Input: part model. Units: mm. Frame: model coordinates. A direction names the side the tool comes from. Round coordinates to 2 decimals unless told otherwise and drop trailing zeros. Loops run counter-clockwise (first coordinate to the right, second up) from the corner with the lowest first, then second, coordinate; pieces in that order, holes last. Notation, with made-up numbers: (51, 6.5) -> (76, 6.5) arc R19 cw to (76, 28.5) -> close; hole circle Ø5 at (66, 22). An arc over 180 degrees is marked (long way). Answer in a Markdown table with one row per item. Add a question column.
Q1. Reachability of faces 5 (the face through (0, -14, 7.7)), 6 (the face through (0, -5.76, 7)), 7 (the face through (7, 15.24, 7)), 8 (the face through (19, -13.502, 5)), 9 (the face through (-19, 1.102, 5)) from +Z, -Z, +X, -X, +Y, -Y: full face, straight path, thin tool, end or side. Return the list, or none.
Q2. Section D-D, the plane z = 11. Output: boundary loops of the cut face in (x, y), and give its area (3 significant figures).
Q3. Section A-A, the plane x = 22. Output: boundary loops of the cut face in (y, z), and give its area (3 significant figures).
Q4. Ray query, L1, parallel to X at y = 1.5, z = 3.75; L2, parallel to Y at x = -22, z = 1.25; L3, parallel to X at y = -10.5, z = 6.75. Return the intervals inside material, ascending. Write a range as from..to.
Q5. Pin query (flat end, axial travel): pin 1 (3 mm diameter, centred on x = 19.5, z = 6, fed in from +Y); pin 2 (6.5 mm diameter, centred on x = 22, z = 6, fed in from -Y); pin 3 (0.7 mm diameter, centred on y = 15.5, z = 7.5, fed in from -X); pin 4 (2.5 mm diameter, centred on x = 22, y = 17, fed in from +Z). Return the tip coordinate at first contact, or that it passes through.
Q6. Mould query, pull axis X, two halves, no side actions, for faces 1 (the face through (4.5, 16, 7)), 2 (the face through (-19, -13.502, 5)), 3 (the face through (13.5, 7, 5)), 4 (the face through (6.2, -14, 5)). Classes: pulls with the +X half, pulls with the -X half, needs draft (parallel to the pull), parting line crosses it, or undercut.
Q7. Section C-C, the plane y = -17. Output: boundary loops of the cut face in (x, z).
Q8. Section B-B, the plane z = 4.25. Output: boundary loops of the cut face in (x, y), and give its area (3 significant figures).
Autodesk Inventor part; units mm, degrees
ref_plane "YZ Plane" through (0, 0, 0) normal (1, 0, 0) x (0, 1, 0)
ref_plane "XZ Plane" through (0, 0, 0) normal (0, 1, 0) x (-1, 0, 0)
ref_plane "XY Plane" through (0, 0, 0) normal (0, 0, 1) x (1, 0, 0)
sketch "スケッチ1" plane through (0, 0, 0) normal (0, 0, 1) x (1, 0, 0)
  line L0 (-25, -20) -> (25, -20)
  line L1 (25, -20) -> (25, 20)
  line L2 (25, 20) -> (-25, 20)
  line L3 (-25, 20) -> (-25, -20)
  line L4 (-25, -20) -> (25, 20) construction
  line L5 (25, -20) -> (-25, 20) construction
  line L6 (-22, -17) -> (22, -17) construction
  line L7 (22, -17) -> (22, 17) construction
  line L8 (22, 17) -> (-22, 17) construction
  line L9 (-22, 17) -> (-22, -17) construction
  line L10 (-22, -17) -> (22, 17) construction
  line L11 (22, -17) -> (-22, 17) construction
  circle A0 centre (-22, -17) radius 1.6
  circle A1 centre (-22, 17) radius 1.6
  circle A2 centre (22, -17) radius 1.6
  circle A3 centre (22, 17) radius 1.6
  line L12 (-25, -13.5025) -> (-13.5, -13.5025)
  line L13 (-13.5, -13.5025) -> (-13.5, -1.1025)
  line L14 (-13.5, -1.1025) -> (-25, -1.1025)
  line L15 (-6.2, -20) -> (-6.2, -8.5)
  line L16 (-6.2, -8.5) -> (6.2, -8.5)
  line L17 (6.2, -8.5) -> (6.2, -20)
  line L18 (-25, 0) -> (25, 0) construction
  line L19 (0, -20) -> (0, 20) construction
  line L20 (-25, 13.5025) -> (-13.5, 13.5025)
  line L21 (-13.5, 13.5025) -> (-13.5, 1.1025)
  line L22 (-13.5, 1.1025) -> (-25, 1.1025)
  line L23 (25, -13.5025) -> (13.5, -13.5025)
  line L24 (13.5, -13.5025) -> (13.5, -1.1025)
  line L25 (13.5, -1.1025) -> (25, -1.1025)
  line L26 (13.5, 1.1025) -> (25, 1.1025)
  line L27 (13.5, 13.5025) -> (13.5, 1.1025)
  line L28 (25, 13.5025) -> (13.5, 13.5025)
  line L29 (-8.75, -5.76) -> (8.75, -5.76)
  line L30 (8.75, -5.76) -> (8.75, 15.24)
  line L31 (8.75, 15.24) -> (-8.75, 15.24)
  line L32 (-8.75, 15.24) -> (-8.75, -5.76)
  line L33 (-8.75, -5.76) -> (8.75, 15.24) construction
  line L34 (8.75, -5.76) -> (-8.75, 15.24) construction
  line L35 (-4.5, 15.24) -> (-4.5, 16.664)
  line L36 (-4.5, 16.664) -> (4.5, 16.664)
  line L37 (4.5, 16.664) -> (4.5, 15.24)
  point P0 (0, 0)
  point P1 (-13.5, -7.3025)
  point P2 (0, -8.5)
  point P3 (0, 4.74)
  point P4 (0, 16.664)
  point P5 (0, 4.74)
  dimension "d0" = 50
  dimension "d1" = 40
  dimension "d2" = 44
  dimension "d3" = 34
  dimension "d4" = 3.2
  dimension "d5" = 3.2
  dimension "d6" = 3.2
  dimension "d7" = 3.2
  dimension "d8" = 11.5
  dimension "d9" = 12.4
  dimension "d10" = 7.3025
  dimension "d11" = 11.5
  dimension "d12" = 12.4
  dimension "d17" = 17.5
  dimension "d18" = 21
  dimension "d19" = 9
  dimension "d20" = 1.424
  dimension "d21" = 15.26
extrude "押し出し1" add sketch "スケッチ1" along normal blind 1.6 contours L3 L12 L13 L14 L22 L21 L20 L2 L1 L28 L27 L26 L25 L24 L23 L0 L17 L16 L15 | L15 L16 L17 L0 | L3 L14 L13 L12 | L3 L20 L21 L22 | L23 L24 L25 L1 | L26 L27 L28 L1 | L32 L31 L30 L29 | L35 L36 L37 L31
extrude "押し出し2" add sketch "スケッチ1" along normal blind 7.7 contours L15 L16 L17 L0 | L3 L14 L13 L12 | L3 L20 L21 L22 | L23 L24 L25 L1 | L26 L27 L28 L1
extrude "押し出し3" add sketch "スケッチ1" along normal blind 12.6 contours L32 L31 L30 L29 | L35 L36 L37 L31
equation "\"d5\" = d4"
equation "\"d6\" = d4"
equation "\"d7\" = d4"
equation "\"d11\" = d8"
equation "\"d12\" = d9"
properties part number "Quad-Load-Cell-Amplifier-to-RS-485-Conv-Module"
Answer block:
| question | item | result |
|---|---|---|
| 1 | face 5 | +Z, +X, -X, -Y |
| 1 | face 6 | +Z |
| 1 | face 7 | +Z, +X, +Y |
| 1 | face 8 | +Z, +X, -Y |
| 1 | face 9 | +Z, -X |
| 2 | outline | (-8.75, -5.76) -> (8.75, -5.76) -> (8.75, 15.24) -> (4.5, 15.24) -> (4.5, 16.66) -> (-4.5, 16.66) -> (-4.5, 15.24) -> (-8.75, 15.24) -> close |
| 2 | area | 380 mm^2 |
| 3 | outline | (-20, 0) -> (-18.6, 0) -> (-18.6, 1.6) -> (-20, 1.6) -> close; (-15.4, 0) -> (15.4, 0) -> (15.4, 1.6) -> (13.5, 1.6) -> (13.5, 7.7) -> (1.1, 7.7) -> (1.1, 1.6) -> (-1.1, 1.6) -> (-1.1, 7.7) -> (-13.5, 7.7) -> (-13.5, 1.6) -> (-15.4, 1.6) -> close; (18.6, 0) -> (20, 0) -> (20, 1.6) -> (18.6, 1.6) -> close |
| 3 | area | 205 mm^2 |
| 4 | L1 | -25..-13.5, -8.75..8.75, 13.5..25 |
| 4 | L2 | -20..-18.6, -15.4..15.4, 18.6..20 |
| 4 | L3 | -25..-13.5, -6.2..6.2, 13.5..25 |
| 5 | pin 1 | y = 13.5 |
| 5 | pin 2 | y = -13.5 |
| 5 | pin 3 | x = -8.75 |
| 5 | pin 4 | through |
| 6 | face 1 | pulls with the +X half |
| 6 | face 2 | needs draft |
| 6 | face 3 | undercut |
| 6 | face 4 | undercut |
| 7 | outline | (-25, 0) -> (-23.6, 0) -> (-23.6, 1.6) -> (-25, 1.6) -> close; (-20.4, 0) -> (20.4, 0) -> (20.4, 1.6) -> (6.2, 1.6) -> (6.2, 7.7) -> (-6.2, 7.7) -> (-6.2, 1.6) -> (-20.4, 1.6) -> close; (23.6, 0) -> (25, 0) -> (25, 1.6) -> (23.6, 1.6) -> close |
| 8 | outline | (-25, -13.5) -> (-13.5, -13.5) -> (-13.5, -1.1) -> (-25, -1.1) -> close; (-25, 1.1) -> (-13.5, 1.1) -> (-13.5, 13.5) -> (-25, 13.5) -> close; (-8.75, -5.76) -> (8.75, -5.76) -> (8.75, 15.24) -> (4.5, 15.24) -> (4.5, 16.66) -> (-4.5, 16.66) -> (-4.5, 15.24) -> (-8.75, 15.24) -> close; (-6.2, -20) -> (6.2, -20) -> (6.2, -8.5) -> (-6.2, -8.5) -> close; (13.5, -13.5) -> (25, -13.5) -> (25, -1.1) -> (13.5, -1.1) -> close; (13.5, 1.1) -> (25, 1.1) -> (25, 13.5) -> (13.5, 13.5) -> close |
| 8 | area | 1,090 mm^2 |
